from build123d import *

# Parameters (mm, degrees)
F0_W     = 152.4
F0_H     = 406.4
F0_R     = 19.05
F1_DEPTH = 12.7
F2_W     = 114.3
F2_H     = 406.4
F3_DEPTH = 12.7
F5_W     = 165.1
F5_H     = 406.4
F5_R     = 19.05
F6_DEPTH = 12.7


with BuildPart() as f1:
    # F0 (on Right) → F1 (new body)
    with BuildSketch(Plane.YZ):
        Rectangle(F0_W, F0_H)
        with Locations((0, -101.6)):
            Circle(F0_R, mode=Mode.SUBTRACT)
        with Locations((0, 101.6)):
            Circle(F0_R, mode=Mode.SUBTRACT)
    extrude(amount=F1_DEPTH)

    # F2 (on face) → F3 (join)
    with BuildSketch(Plane(origin=(0, 76.2, 0), x_dir=(-1, 0, 0), z_dir=(0, 1, 0))):
        with Locations((-57.15, 0)):
            Rectangle(F2_W, F2_H)
    extrude(amount=F3_DEPTH)

    # F5 (on face) → F6 (join)
    with BuildSketch(Plane.YZ.offset(114.3)):
        with Locations((6.35, 0)):
            Rectangle(F5_W, F5_H)
        with Locations((0, -101.6)):
            Circle(F5_R, mode=Mode.SUBTRACT)
        with Locations((0, 101.6)):
            Circle(F5_R, mode=Mode.SUBTRACT)
    extrude(amount=F6_DEPTH)


solid = f1.part
Input: part model. Units: mm. Frame: model coordinates. A direction names the side the tool comes from. Give positions to 0.01 mm unless a question says otherwise; leave off trailing zeros. Write each loop counter-clockwise with the first axis right and the second up, starting at its lowest first coordinate (ties: lowest second). Pieces come first, ordered by that corner, then holes. Notation, with made-up numbers: M 20,48.25 L 53,48.25 A28 ccw 53,76.25 Z; hole C 59.5,-26 d9. An arc over 180 degrees is marked long. Write item = value, one per line. Start each with the question number.
1) Draft query along X for faces 3 (the cylindrical face through (120.561, -2.48, -82.712)), 4 (the flat face through (0, 5, -3)), 5 (the flat face through (127, 5, 3)), 6 (the flat face through (114.3, -1, 3)). Return one class per face: +X half, -X half, draft (parallel to the pull), parting line (faces both ways), or undercut.
2) Cut plane B-B on z = 101.6. Return the cut outline in (x, y), then the cut area to 3 significant figures.
3) Cut plane C-C on y = -62.5. Return the cut outline in (x, z).
4) Material intervals for line 1 along Z through (x, y) = (119.25, 0); line 2 along X through (y, z) = (50, -60.5); line 3 along Y through (x, z) = (9, -101), sorted ascending. Write a range as [from, to].
5) Cut plane A-A on y = 0. Return the cut outline in (x, z), then the cut area to 3 significant figures.
6) Reachability of faces 1 (the flat face through (64, 76.2, 3)), 2 (the cylindrical face through (6.261, -2.48, -82.712)) from +Z, -Z, +X, -X, +Y, -Y: full face, straight path, thin tool, end or side. Return the list, or none.
7) First-contact query: pin 1 Ø10 at (x, z) = (92.5, 134.5) entering from -Y. Flat tip, straight axial feed; report the tip coordinate or a pass-through.
8) Cut plane D-D on x = 118. Return the cut outline in (y, z).
Solved:
q1.face_3 = draft
q1.face_4 = -X half
q1.face_5 = +X half
q1.face_6 = undercut
q2.outline = M 0,-76.2 L 12.7,-76.2 L 12.7,-19.05 L 0,-19.05 Z; M 0,19.05 L 12.7,19.05 L 12.7,76.2 L 114.3,76.2 L 114.3,19.05 L 127,19.05 L 127,88.9 L 0,88.9 Z; M 114.3,-76.2 L 127,-76.2 L 127,-19.05 L 114.3,-19.05 Z
q2.area = 4,520 mm2
q3.outline = M 0,-203.2 L 12.7,-203.2 L 12.7,203.2 L 0,203.2 Z; M 114.3,-203.2 L 127,-203.2 L 127,203.2 L 114.3,203.2 Z
q4.line_1 = [-203.2, -120.65], [-82.55, 82.55], [120.65, 203.2]
q4.line_2 = [0, 12.7], [114.3, 127]
q4.line_3 = [-76.2, -19.04], [19.04, 88.9]
q5.outline = M 0,-203.2 L 12.7,-203.2 L 12.7,-120.65 L 0,-120.65 Z; M 0,-82.55 L 12.7,-82.55 L 12.7,82.55 L 0,82.55 Z; M 0,120.65 L 12.7,120.65 L 12.7,203.2 L 0,203.2 Z; M 114.3,-203.2 L 127,-203.2 L 127,-120.65 L 114.3,-120.65 Z; M 114.3,-82.55 L 127,-82.55 L 127,82.55 L 114.3,82.55 Z; M 114.3,120.65 L 127,120.65 L 127,203.2 L 114.3,203.2 Z
q5.area = 8,390 mm2
q6.face_1 = +Z, -Z, -Y
q6.face_2 = +X, -X
q7.pin_1 = 76.2
q8.outline = M -76.2,-203.2 L 88.9,-203.2 L 88.9,203.2 L -76.2,203.2 Z; hole C 0,-101.6 d38.1; hole C 0,101.6 d38.1
